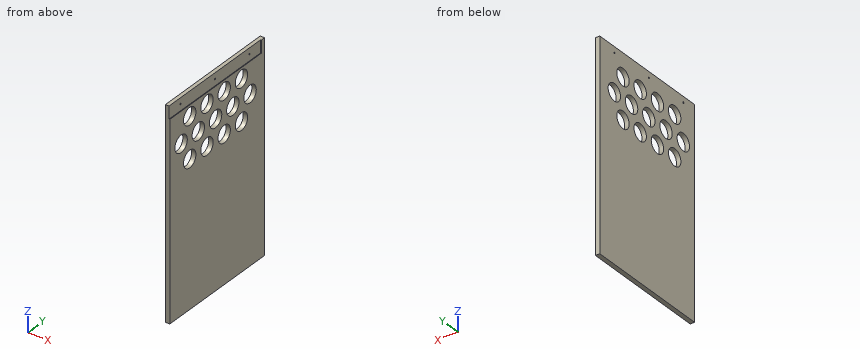
```python
from build123d import *

# Parameters (mm, degrees)
F0_W     = 19.05
F0_H     = 337.82
F1_DEPTH = 539.75
F2_R     = 36.5125
F3_DEPTH = 25.4
F4_DEPTH = 557.53
F5_DEPTH = 19.05
F6_W     = 3.175
F6_H     = 53.975
F7_DEPTH = 539.75
F9_D     = 6.5278


# Not quite as in the source:
# - a feature names something its author has since deleted; it is built from what else it names


with BuildPart() as f1:
    # F0 (on Front) → F1 (new body)
    with BuildSketch(Plane.XZ):
        Rectangle(F0_W, F0_H)
    extrude(amount=F1_DEPTH)

    # F2 (on face) → F3 (cut)
    with BuildSketch(Plane.YZ.offset(9.525)):
        with Locations((-269.875, -19.05)):
            Circle(F2_R)
        with Locations((-320.6515127996, 68.8975)):
            Circle(F2_R)
        with Locations((-219.0515127996, 68.8975)):
            Circle(F2_R)
        with Locations((-168.275, -19.05)):
            Circle(F2_R)
        with Locations((-117.4515127996, 68.8975)):
            Circle(F2_R)
        with Locations((-66.675, -19.05)):
            Circle(F2_R)
        with Locations((-371.475, -19.05)):
            Circle(F2_R)
        with Locations((-422.2984872004, 68.8975)):
            Circle(F2_R)
        with Locations((-473.075, -19.05)):
            Circle(F2_R)
        with Locations((-422.2984872004, -106.9975)):
            Circle(F2_R)
        with Locations((-320.6515127996, -106.9975)):
            Circle(F2_R)
        with Locations((-219.0515127996, -106.9975)):
            Circle(F2_R)
        with Locations((-117.4515127996, -106.9975)):
            Circle(F2_R)
    extrude(amount=-F3_DEPTH, mode=Mode.SUBTRACT)

    # F4 (add): a face of the model
    f4_faces = [f1.faces().sort_by_distance(p)[0] for p in [
        (0, -269.875, -168.91),
    ]]
    extrude(f4_faces, amount=F4_DEPTH)

    # F5 (add): a face of the model
    f5_faces = [f1.faces().sort_by_distance(p)[0] for p in [
        (0, 0, -278.765),
    ]]
    extrude(f5_faces, amount=F5_DEPTH)

    # F6 (on face) → F7 (cut, through all)
    with BuildSketch(Plane.XZ.offset(539.75)):
        with Locations((7.9375, 141.9225)):
            Rectangle(F6_W, F6_H)
    extrude(amount=-F7_DEPTH, mode=Mode.SUBTRACT)

    # F9 (through all)
    with Locations(Plane(origin=(-9.525, 0, 0), x_dir=(0, -1, 0), z_dir=(-1, 0, 0))):
        with Locations((66.675, 143.51), (269.875, 143.51), (473.075, 143.51)):
            Hole(F9_D / 2)


solid = f1.part
```
The listing builds one solid part. Answer for the finished solid, in the listing's coordinates (mm). Give positions to 0.01 mm unless a question says otherwise; leave off trailing zeros. Loops run counter-clockwise (first coordinate to the right, second up) from the corner with the lowest first, then second, coordinate; pieces in that order, holes last. Notation, with made-up numbers: (65, 17) - (94, 17) arc R7 cw to (94, 21) - close; hole circle Ø8 at (52, 81.25). An arc over 180 degrees is marked (long way). Return JSON: item names as keys, results as strings. Group by question number.
1. Find section C-C (z = -121). Write down the section's boundary in (x, y) (3 decimals), then the cut area to 3 significant figures.
2. Given pin 1 Ø5 at (y, z) = (-66.675, 143.51) entering from -X; pin 2 Ø16 at (y, z) = (-223.5, 146.5) entering from +X; pin 3 Ø3.5 at (x, z) = (8.5, 141.5) entering from -Y, each flat-ended and moving along its own axis, determine where each tip first touches the part or whether it passes through.
3. Straight lines are drawn through the part: line 1 (Z direction, x = -2.5, y = -66); line 2 (Y direction, x = -5.25, z = 143.51); line 3 (Z direction, x = -6.25, y = -420). For each, find the intervals that lie inside material, in ascending order. Write a range as [from, to].
4. Find section B-B (y = -495). Write down the section's boundary in (x, z) (3 decimals).
5. Find section A-A (z = -19.05). State how many separate pieces and enclosed holes the cut face has, then the cut area to 3 significant figures.
Verdict:
{
 "1": {"outline": "(-9.525, -539.75) - (9.525, -539.75) - (9.525, -456.019) - (-9.525, -456.019) - close; (-9.525, -388.578) - (9.525, -388.578) - (9.525, -354.372) - (-9.525, -354.372) - close; (-9.525, -286.931) - (9.525, -286.931) - (9.525, -252.772) - (-9.525, -252.772) - close; (-9.525, -185.331) - (9.525, -185.331) - (9.525, -151.172) - (-9.525, -151.172) - close; (-9.525, -83.731) - (9.525, -83.731) - (9.525, 19.05) - (-9.525, 19.05) - close", "area": "5,510 mm^2"},
 "2": {"pin 1": "passes through", "pin 2": "stops at x = 6.35", "pin 3": "stops at y = 0"},
 "3": {"line 1": "z = [-726.44, -55.56], [17.46, 140.32], [146.7, 168.91]", "line 2": "y = [-539.75, -476.34], [-469.81, -273.14], [-266.61, -69.94], [-63.41, 19.05]", "line 3": "z = [-726.44, -143.44], [-70.56, 32.46], [105.34, 168.91]"},
 "4": {"outline": "(-9.525, -726.44) - (9.525, -726.44) - (9.525, -48.247) - (-9.525, -48.247) - close; (-9.525, 10.147) - (9.525, 10.147) - (9.525, 114.935) - (6.35, 114.935) - (6.35, 168.91) - (-9.525, 168.91) - close"},
 "5": {"separate pieces": "6", "enclosed holes": "0", "area": "3,690 mm^2"}
}
